Study the drawing (mm; zero at the part's minimum x, y, z) and answer. A direction names the side the tool comes from. Coordinates: 2 decimals unless noted, no trailing zeros. Write each loop counter-clockwise with the first axis right and the second up, starting at its lowest first coordinate (ties: lowest second). Pieces come first, ordered by that corner, then holes. Notation, with made-up numbers: M -26,6.5 L 18,6.5 A26 ccw 18,26.5 Z; hole C 20,17.25 d2. An arc over 180 degrees is marked long. Answer as a JSON object with one key per item and string values. Group by question number.
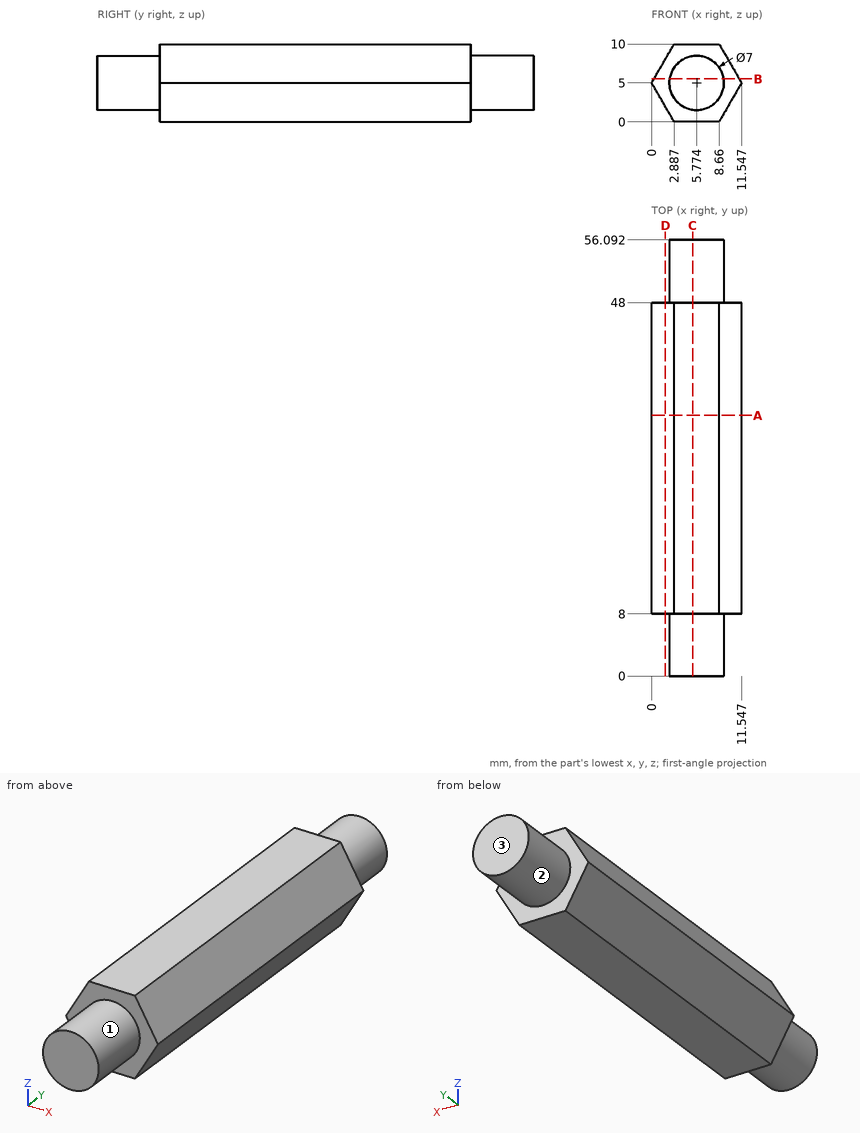
Item 1: A cutting plane is placed at C-C, the plane x = 5.25. Write down the section's boundary in (y, z).
Item 2: A cutting plane is placed at D-D, the plane x = 1.75. Write down the section's boundary in (y, z).
Item 3: A cutting plane is placed at A-A, the plane y = 33.5. Write down the section's boundary in (x, z), and give its area (3 significant figures).
Item 4: A flat-ended cylindrical pin translates along its axis: pin 1 Ø6 at (y, z) = (18.5, 5.5) entering from -X. Find the tip coordinate at first contact, or state that the pin passes through.
Item 5: A cutting plane is placed at B-B, the plane z = 5.5. Write down the section's boundary in (x, y), and give its area (3 significant figures).
Item 6: A tool of negligible diameter and unlimited length cuts with its end or side. For the marked faces 1, 2 and 3, from which of +Z, -Z, +X, -X, +Y, -Y can it reach the whole face along a straight path? Write none if from no direction.
Item 7: Consider L1, parallel to Y at x = 8.5, z = 8; L2, parallel to X at y = 33.5, z = 7.5 (1 decimal); L3, parallel to Z at x = 2.75, y = 9.5 (1 decimal). Determine where each line is inside the solid, lowest interval first. Write a range as from..to.
Answer:
{
 "1": {"outline": "M 0,1.54 L 8,1.54 L 8,0 L 48,0 L 48,1.54 L 56.09,1.54 L 56.09,8.46 L 48,8.46 L 48,10 L 8,10 L 8,8.46 L 0,8.46 Z"},
 "2": {"outline": "M 8,1.97 L 48,1.97 L 48,8.03 L 8,8.03 Z"},
 "3": {"outline": "M 0,5 L 2.89,0 L 8.66,0 L 11.55,5 L 8.66,10 L 2.89,10 Z", "area": "86.6 mm2"},
 "4": {"pin 1": "x = 0"},
 "5": {"outline": "M 0.29,8 L 2.31,8 L 2.31,0 L 9.24,0 L 9.24,8 L 11.26,8 L 11.26,48 L 9.24,48 L 9.24,56.09 L 2.31,56.09 L 2.31,48 L 0.29,48 Z", "area": "550 mm2"},
 "6": {"face 1": "-Y", "face 2": "+Y", "face 3": "+Z, -Z, +X, -X, +Y"},
 "7": {"L1": "8..48", "L2": "1.4..10.1", "L3": "0.2..9.8"}
}
